Source: CAD feature listing. Evaluate the final solid. Frame: model axes, mm. Face numbers are marked on the shaded views. Coordinates: 2 decimals unless noted, no trailing zeros. Order: outer loops, then holes, each group sorted by start corner. A loop starts at its lowest first (then second) coordinate and runs counter-clockwise, first axis right, second up.
```python
from build123d import *

# Parameters (mm, degrees)
F2_W     = 4.486534
F2_H     = 0.762
F3_DEPTH = 30.862
F4_W     = 50.8
F4_H     = 25.4
F5_DEPTH = 0.508


with BuildPart() as f1:
    # F0 (on Front) → F1 (revolve)
    with BuildSketch(Plane.XZ):
        Polygon((0, 3.683), (0, 2.667), (9.525, 2.667), (9.525, 2.032), (30.861, 2.032), (30.861, 3.257631), (29.2735, 3.683), align=None)
    revolve(axis=Axis((17.153487, 0, 0), (1, 0, 0)))

    # F2 (on face) → F3 (cut, through all)
    with BuildSketch(Plane(origin=(0, 0, 0), x_dir=(0, -1, 0), z_dir=(-1, 0, 0))):
        with Locations((0, -3.302)):
            Rectangle(F2_W, F2_H)
    extrude(amount=-F3_DEPTH, mode=Mode.SUBTRACT)

    # F4 (on face) → F5 (join)
    with BuildSketch(Plane(origin=(0, 0, -2.921), x_dir=(1, 0, 0), z_dir=(0, 0, -1))):
        with Locations((14.63675, 0)):
            Rectangle(F4_W, F4_H)
    extrude(amount=F5_DEPTH)


solid = f1.part
```
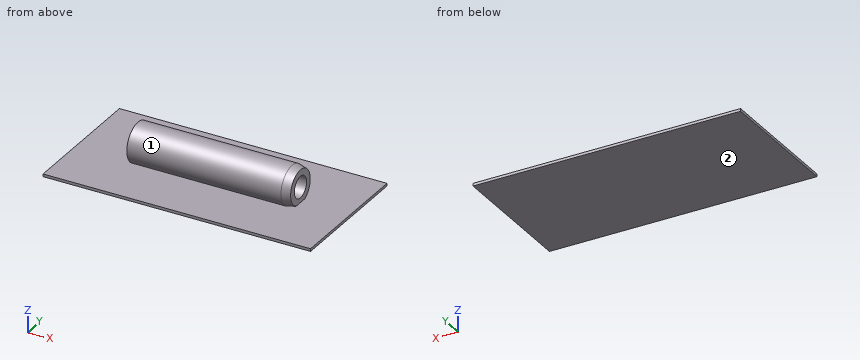
1. Section query A-A on z = 0. Return loops of the section in (x, y) (1 decimal), plus the area to 3 significant figures.
Findings:
outline: (0, -3.7) - (29.3, -3.7) - (30.9, -3.3) - (30.9, -2) - (9.5, -2) - (9.5, -2.7) - (0, -2.7) - close; (0, 2.7) - (9.5, 2.7) - (9.5, 2) - (30.9, 2) - (30.9, 3.3) - (29.3, 3.7) - (0, 3.7) - close
area: 89.1 mm2
2. Section query C-C on x = 20.5. Return loops of the section in (y, z).
Findings:
outline: (-12.7, -3.43) - (12.7, -3.43) - (12.7, -2.92) - (2.24, -2.92) arc R3.68 ccw (long way) to (-2.24, -2.92) - (-12.7, -2.92) - close; hole circle Ø4.06 at (0, 0)
3. Pin query (flat end, axial travel): P1, Ø6, axis at x = 21.5, y = -5, coming from the +Z side; P2, Ø4, axis at x = 0.5, z = 3, coming from the +Y side; P3, Ø3, axis at y = -6, z = 0.5, coming from the -X side; P4, Ø2, axis at x = 14.5, z = -1.5, coming from the +Y side. Return the tip coordinate at first contact, or that it passes through.
Findings:
P1: stops at z = 3.09
P2: stops at y = 3.54
P3: passes through
P4: stops at y = 3.65
4. Section query D-D on y = 9.25. Return loops of the section in (x, z).
Findings:
outline: (-10.76, -3.43) - (40.04, -3.43) - (40.04, -2.92) - (-10.76, -2.92) - close
5. Ray query, line 1 (Z direction, x = 15.25, y = 0); line 2 (Z direction, x = 4.5, y = 0); line 3 (Y direction, x = 23.5, z = 0). Return the intervals inside material, ascending.
Findings:
line 1: z = -3.43 to -2.03, 2.03 to 3.68
line 2: z = -3.43 to -2.67, 2.67 to 3.68
line 3: y = -3.68 to -2.03, 2.03 to 3.68
6. Draft query along Z for the marked faces 1 and 2. Return one class per face: released by +Z, released by -Z, zero draft, split by the parting line, or undercut.
Findings:
face 1: undercut
face 2: released by -Z
